from build123d import *

# Parameters (mm, degrees)
SKETCH_1_W                   = 414
SKETCH_1_H                   = 82
EXTRUDE_1_DEPTH              = 12
SKETCH_2_R                   = 6
SKETCH_2_R_2                 = 12
SKETCH_2_W                   = 27.5
SKETCH_2_H                   = 31.5
CUT_EXTRUDE_5_DEPTH          = 13
FILLET_1_R                   = 3
HOLE_WIZARD_M3_1_D           = 2.5
HOLE_WIZARD_M3_1_CSINK_D     = 3.05
HOLE_WIZARD_M3_1_CSINK_ANGLE = 90
HOLE_WIZARD_M4_1_D           = 3.3
HOLE_WIZARD_M4_1_CSINK_D     = 4.05
HOLE_WIZARD_M4_1_CSINK_ANGLE = 90
HOLE_WIZARD_M4_3_D           = 3.3
HOLE_WIZARD_M4_3_DEPTH       = 7.1
HOLE_WIZARD_M4_3_CSINK_D     = 4.05
HOLE_WIZARD_M4_3_CSINK_ANGLE = 90
HOLE_WIZARD_M4_3_TIP         = 0.991420021
HOLE_WIZARD_M4_4_D           = 3.3
HOLE_WIZARD_M4_4_DEPTH       = 7.1
HOLE_WIZARD_M4_4_CSINK_D     = 4.05
HOLE_WIZARD_M4_4_CSINK_ANGLE = 90
HOLE_WIZARD_M4_4_TIP         = 0.991420021


with BuildPart() as part:
    # 草圖1 → 填料-伸長1 (new body)
    with BuildSketch(Plane.XY):
        with Locations((207, 41)):
            Rectangle(SKETCH_1_W, SKETCH_1_H)
    extrude(amount=EXTRUDE_1_DEPTH)

    # 草圖2 → 除料-伸長5 (cut, through all)
    with BuildSketch(Plane.XY):
        with Locations((130, 56)):
            Circle(SKETCH_2_R)
        with Locations((130, 26)):
            Circle(SKETCH_2_R)
        with Locations((284, 56)):
            Circle(SKETCH_2_R)
        with Locations((284, 26)):
            Circle(SKETCH_2_R)
        with Locations((50, 41)):
            Circle(SKETCH_2_R_2)
        with Locations((364, 41)):
            Circle(SKETCH_2_R_2)
        with Locations((207, 25.25)):
            Rectangle(SKETCH_2_W, SKETCH_2_H)
    extrude(amount=CUT_EXTRUDE_5_DEPTH, mode=Mode.SUBTRACT)

    # 圓角1
    fillet_1_edges = [part.edges().sort_by_distance(p)[0] for p in [
        (220.75, 9.5, 6),
        (220.75, 41, 6),
        (193.25, 41, 6),
        (193.25, 9.5, 6),
    ]]
    fillet(fillet_1_edges, radius=FILLET_1_R)

    # M3 螺紋孔1 (through all)
    with Locations(Plane(origin=(0, 0, 0), x_dir=(1, 0, 0), z_dir=(0, 0, -1))):
        with Locations((59.5, -53), (40.5, -29), (189, -25.25), (225, -25.25), (373.5, -53), (354.5, -29)):
            CounterSinkHole(HOLE_WIZARD_M3_1_D / 2, HOLE_WIZARD_M3_1_CSINK_D / 2, counter_sink_angle=HOLE_WIZARD_M3_1_CSINK_ANGLE)

    # M4 螺紋孔1 (through all)
    with Locations(Plane(origin=(0, 82, 0), x_dir=(1, 0, 0), z_dir=(0, 1, 0))):
        with Locations((21, -7), (145, -7), (269, -7), (393, -7)):
            CounterSinkHole(HOLE_WIZARD_M4_1_D / 2, HOLE_WIZARD_M4_1_CSINK_D / 2, counter_sink_angle=HOLE_WIZARD_M4_1_CSINK_ANGLE)

    # M4 螺紋孔3
    with Locations(Plane(origin=(414, 0, 0), x_dir=(0, 0, -1), z_dir=(1, 0, 0))):
        with Locations((-7, 16), (-7, 66)):
            CounterSinkHole(HOLE_WIZARD_M4_3_D / 2, HOLE_WIZARD_M4_3_CSINK_D / 2, depth=HOLE_WIZARD_M4_3_DEPTH, counter_sink_angle=HOLE_WIZARD_M4_3_CSINK_ANGLE)
            with Locations((0, 0, -(HOLE_WIZARD_M4_3_DEPTH + HOLE_WIZARD_M4_3_TIP / 2))):  # 118° drill point
                Cone(0, HOLE_WIZARD_M4_3_D / 2, HOLE_WIZARD_M4_3_TIP, mode=Mode.SUBTRACT)

    # M4 螺紋孔4
    with Locations(Plane.ZY):
        with Locations((7, 16), (7, 66)):
            CounterSinkHole(HOLE_WIZARD_M4_4_D / 2, HOLE_WIZARD_M4_4_CSINK_D / 2, depth=HOLE_WIZARD_M4_4_DEPTH, counter_sink_angle=HOLE_WIZARD_M4_4_CSINK_ANGLE)
            with Locations((0, 0, -(HOLE_WIZARD_M4_4_DEPTH + HOLE_WIZARD_M4_4_TIP / 2))):  # 118° drill point
                Cone(0, HOLE_WIZARD_M4_4_D / 2, HOLE_WIZARD_M4_4_TIP, mode=Mode.SUBTRACT)


solid = part.part
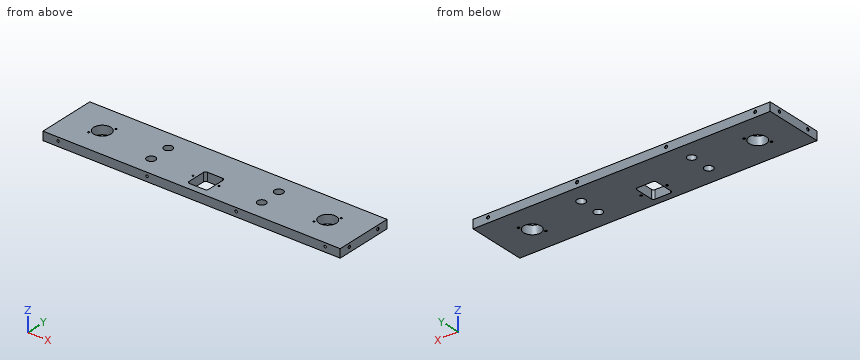
Could you check a few things on this model? Use its own coordinates, in mm. Give positions to 0.01 mm unless a question says otherwise; leave off trailing zeros. Order: outer loops, then holes, each group sorted by start corner. A loop starts at its lowest first (then second) coordinate and runs counter-clockwise, first axis right, second up.
1. Suppose I cut it at A-A (x = 284). Write out the boundary of the cut face in (y, z).
Answers below:
outline: (0, 0) - (20, 0) - (20, 12) - (0, 12) - close; (32, 0) - (50, 0) - (50, 12) - (32, 12) - close; (62, 0) - (82, 0) - (82, 12) - (62, 12) - close
2. I need wall thicknesses on L1, parallel to Y at x = 130, z = 2.75; L2, parallel to Y at x = 409.5, z = 7; L3, parallel to X at y = 56, z = 9.25. Which ranges of each line are inside material? Lowest first, please.
Answers below:
L1: y = 0 to 20, 32 to 50, 62 to 82
L2: y = 0 to 14.35, 17.65 to 64.35, 67.65 to 82
L3: x = 0 to 124, 136 to 278, 290 to 414
3. For pin 1 (3 mm diameter, centred on x = 354.5, y = 29, fed in from -Z) (3 decimals); pin 2 (2 mm diameter, centred on y = 66, z = 7, fed in from -X), each with a flat end and sliding along its axis, tell me the tip position at first contact or that it passes through.
Answers below:
pin 1: stops at z = 0.025
pin 2: stops at x = 7.49
4. Suppose I cut it at B-B (z = 3). State how many separate pieces and enclosed holes the cut face has, plus the area to 3 significant figures.
Answers below:
separate pieces: 1
enclosed holes: 13
area: 31,700 mm2
